Source: CAD feature listing. Evaluate the final solid. Frame: model axes, mm. A direction names the side the tool comes from. Coordinates: 2 decimals unless noted, no trailing zeros. Write each loop counter-clockwise with the first axis right and the second up, starting at its lowest first coordinate (ties: lowest second). Pieces come first, ordered by that corner, then holes. Notation, with made-up numbers: M 41,-36.5 L 66,-36.5 A18 ccw 66,-1.5 Z; hole C 38.5,62 d11. An arc over 180 degrees is marked long. Write item = value, one per line. Start each with the question number.
1. Access query for faces 1 (the face through (-9.65, 2.03, 2.3)), 2 (the face through (2.8, 7, 0)), 3 (the face through (6.5, -0.25, 6.37)), 4 (the face through (6.6, 0, -6.6)). Directions: +Z, -Z, +X, -X, +Y, -Y. A direction counts if a zero-diameter tool reaches every point of the face in a straight line with its end or side. Return the directions, or none.
2. Section query A-A (z = 0). Give the number of separate pieces and of enclosed holes in the cut face, then the cut area to 3 significant figures.
3. Pin query (flat end, axial travel): pin 1 Ø5 at (x, z) = (-11, 12) entering from -Y; pin 2 Ø5.5 at (x, z) = (12.5, 0) entering from -Y; pin 3 Ø2 at (y, z) = (4, 3.5) entering from -X; pin 4 Ø4 at (x, y) = (-5.5, 4) entering from -Z. Return the tip coordinate at first contact, or that it passes through.
4. Section query C-C (y = 3). Output: boundary loops of the cut face in (x, z).
5. Pull-direction query (Z, two-part tool) for faces 5 (the face through (-6.5, 0, -6.6)), 6 (the face through (2, 6, 13)), 7 (the face through (-7.12, 1.97, 7.02)); classes: pulls with the +Z half, pulls with the -Z half, needs draft (parallel to the pull), parting line crosses it, or undercut.
6. Line query: line 1 along Z through (x, y) = (0, 7.35); line 2 along X through (y, z) = (4.75, 2.5); line 3 along X through (y, z) = (5, -3). Output: solid intervals per line, ascending.
```python
from build123d import *

# Parameters (mm, degrees)
ESQUISSE1_R                  = 10
BOSS_EXTRU_1_DEPTH           = 4
ESQUISSE8_R                  = 11
BOSS_EXTRU_4_DEPTH           = 0.5
ESQUISSE3_R                  = 17.5
ESQUISSE3_R_2                = 1.7
BOSS_EXTRU_2_DEPTH           = 3.5
ENL_V_MAT_EXTRU_2_DEPTH      = 26.154522456
ENL_V_MAT_EXTRU_2_DEPTH_BACK = 1.5
ESQUISSE4_R                  = 3.55
ESQUISSE11_OUTSIDE_W         = 47.028
ESQUISSE11_OUTSIDE_H         = 47.028
ENL_V_MAT_EXTRU_3_DEPTH      = 27.009613607
CONG_1_R                     = 4
CONG_2_R                     = 1
CHANFREIN2_SIZE              = 0.4
ESQUISSE12_R                 = 1.7
ENL_V_MAT_EXTRU_4_DEPTH      = 27.009613773
ESQUISSE13_W                 = 5.6
ESQUISSE13_H                 = 5.6
ENL_V_MAT_EXTRU_5_DEPTH      = 2
BOSS_EXTRU_5_START           = 0.5
ESQUISSE14_R                 = 9.1
ESQUISSE14_R_2               = 1.7
BOSS_EXTRU_5_DEPTH           = 0.5
ESQUISSE15_R                 = 3.55
ENL_V_MAT_EXTRU_6_DEPTH      = 0.5


with BuildPart() as part:
    # Esquisse1 → Boss.-Extru.1 (new body)
    with BuildSketch(Plane(origin=(0, 0, 0), x_dir=(1, 0, 0), z_dir=(0, 1, 0))):
        with Locations(Location((0, 0, 0), (0, 0, 270))):
            Circle(ESQUISSE1_R)
    extrude(amount=BOSS_EXTRU_1_DEPTH)

    # Esquisse8 → Boss.-Extru.4 (add)
    with BuildSketch(Plane(origin=(0, 4, 0), x_dir=(1, 0, 0), z_dir=(0, 1, 0))):
        with Locations(Location((0, 0, 0), (0, 0, 270))):
            Circle(ESQUISSE8_R)
    extrude(amount=BOSS_EXTRU_4_DEPTH)

    # Esquisse3 → Boss.-Extru.2 (add)
    with BuildSketch(Plane(origin=(0, 4.5, 0), x_dir=(1, 0, 0), z_dir=(0, 1, 0))):
        with Locations(Location((0, 0, 0), (0, 0, 270))):
            Circle(ESQUISSE3_R)
        with Locations(Location((-12.5, 0, 0), (0, 0, 26.18008635))):
            Circle(ESQUISSE3_R_2, mode=Mode.SUBTRACT)
        with Locations(Location((0, 12.5, 0), (0, 0, 243.81991365))):
            Circle(ESQUISSE3_R_2, mode=Mode.SUBTRACT)
        with Locations(Location((12.5, 0, 0), (0, 0, 153.81991365))):
            Circle(ESQUISSE3_R_2, mode=Mode.SUBTRACT)
        with Locations(Location((0, -12.5, 0), (0, 0, 116.18008635))):
            Circle(ESQUISSE3_R_2, mode=Mode.SUBTRACT)
    extrude(amount=BOSS_EXTRU_2_DEPTH)

    # Esquisse4 → Enl_v. mat.-Extru.2 (cut, two sides: drawn at the far end of the back side and taken through both)
    with BuildSketch(Plane.XZ.offset(-4.5).offset(-ENL_V_MAT_EXTRU_2_DEPTH_BACK)):
        with Locations(Location((0, -12.5, 0), (0, 0, 129.122124479))):
            Circle(ESQUISSE4_R)
        with Locations(Location((-12.5, 0, 0), (0, 0, 57.371953872))):
            Circle(ESQUISSE4_R)
        with Locations(Location((0, 12.5, 0), (0, 0, 212.628046128))):
            Circle(ESQUISSE4_R)
        with Locations(Location((12.5, 0, 0), (0, 0, 122.628046128))):
            Circle(ESQUISSE4_R)
    extrude(amount=ENL_V_MAT_EXTRU_2_DEPTH + ENL_V_MAT_EXTRU_2_DEPTH_BACK, mode=Mode.SUBTRACT)

    # Esquisse11 outside → Enl_v. mat.-Extru.3 (cut, through all)
    with BuildSketch(Plane(origin=(0, 8, 0), x_dir=(1, 0, 0), z_dir=(0, 1, 0))):
        Rectangle(ESQUISSE11_OUTSIDE_W, ESQUISSE11_OUTSIDE_H)
        with BuildLine():
            ThreePointArc((-5.365249295, -11.29), (0, -18), (5.365249295, -11.29))
            ThreePointArc((5.365249295, -11.29), (8.838834765, -8.838834765), (11.29, -5.365249295))
            ThreePointArc((11.29, -5.365249295), (18, 0), (11.29, 5.365249295))
            ThreePointArc((11.29, 5.365249295), (8.838834765, 8.838834765), (5.365249295, 11.29))
            ThreePointArc((5.365249295, 11.29), (0, 18), (-5.365249295, 11.29))
            ThreePointArc((-5.365249295, 11.29), (-8.838834765, 8.838834765), (-11.29, 5.365249295))
            ThreePointArc((-11.29, 5.365249295), (-18, 0), (-11.29, -5.365249295))
            ThreePointArc((-11.29, -5.365249295), (-8.838834765, -8.838834765), (-5.365249295, -11.29))
        make_face(mode=Mode.SUBTRACT)
    extrude(amount=-ENL_V_MAT_EXTRU_3_DEPTH, mode=Mode.SUBTRACT)

    # Cong_1
    cong_1_edges = [part.edges().sort_by_distance(p)[0] for p in [
        (11.29, 6.25, -5.365249295),
        (5.365249295, 6.25, 11.29),
        (-11.29, 6.25, 5.365249295),
        (-5.365249295, 6.25, -11.29),
        (11.29, 6.25, 5.365249295),
        (-5.365249295, 6.25, 11.29),
        (-11.29, 6.25, -5.365249295),
        (5.365249295, 6.25, -11.29),
        (-2.702942841, 6.25, -17.29),
        (2.702942841, 6.25, -17.29),
        (-17.29, 6.25, 2.702942841),
        (-17.29, 6.25, -2.702942841),
        (2.702942841, 6.25, 17.29),
        (-2.702942841, 6.25, 17.29),
        (17.29, 6.25, -2.702942841),
        (17.29, 6.25, 2.702942841),
    ]]
    fillet(cong_1_edges, radius=CONG_1_R)

    # Cong_2
    # the kernel refuses this fillet: 1 mm, written as the material it takes off along each edge
    with BuildSketch(Plane(origin=(2.239962765, 4, -9.7459), x_dir=(0.968803091142529, 0, 0.24783173846922987), z_dir=(0, -1, 0)), Plane(origin=(-9.7459, 4, -2.239962765), x_dir=(0.24783173846923087, 0, -0.9688030911425286), z_dir=(0, -1, 0)), Plane(origin=(-2.239962765, 4, 9.7459), x_dir=(-0.9688030911425278, 0, -0.24783173846923437), z_dir=(0, -1, 0)), Plane(origin=(9.7459, 4, 2.239962765), x_dir=(-0.24783173846923068, 0, 0.9688030911425288), z_dir=(0, -1, 0))) as cong_2_piece_1:
        with BuildLine():
            CenterArc((0.465994929, 0.999699191), CONG_2_R, 223.166437968, 48.238942041)
            ThreePointArc((-0.263374559, 0.315579209), (-0.127115959, 0.161604715), (0, 0))
            ThreePointArc((0, 0), (0.245260489, -0.003008088), (0.490520978, 0))
        make_face()
    extrude(amount=5.226302444, mode=Mode.SUBTRACT)
    with BuildSketch(Plane(origin=(-2.239962765, 4, -9.7459), x_dir=(0.8110309236137252, 0, 0.5850032828474281), z_dir=(0, -1, 0)), Plane(origin=(9.7459, 4, -2.239962765), x_dir=(-0.5850032828485626, 0, 0.8110309236129067), z_dir=(0, -1, 0))) as cong_2_piece_2:
        with BuildLine():
            CenterArc((0.468936447, 0.998322771), CONG_2_R, 218.44215541, 48.238942041)
            ThreePointArc((-0.314299789, 0.376598556), (-0.15945936, 0.186371855), (0, 0))
            ThreePointArc((0, 0), (0.205521529, 0.005954162), (0.411043058, 0))
        make_face()
    extrude(amount=5.226302444, mode=Mode.SUBTRACT)
    with BuildSketch(Plane(origin=(-9.7459, 4, 2.239962765), x_dir=(0.2478317384692303, 0, 0.9688030911425288), z_dir=(0, -1, 0)), Plane(origin=(2.239962765, 4, 9.7459), x_dir=(0.9688030911425286, 0, -0.2478317384692314), z_dir=(0, -1, 0))) as cong_2_piece_3:
        with BuildLine():
            CenterArc((0.465994929, -0.999699191), CONG_2_R, 88.594619991, 48.238942041)
            ThreePointArc((-0.263374559, -0.315579209), (-0.127115959, -0.161604715), (0, 0))
            ThreePointArc((0, 0), (0.245260489, 0.003008088), (0.490520978, 0))
        make_face()
    extrude(amount=5.226302444, mode=Mode.SUBTRACT)

    # Chanfrein2
    chanfrein2_edges = [part.edges().sort_by_distance(p)[0] for p in [
        (-14.627830223, 8, -5.071719486),
        (8.838834765, 8, 8.838834765),
        (14.627830223, 8, 5.071719486),
        (17.5, 8, 0),
        (14.627830223, 8, -5.071719486),
        (8.838834765, 8, -8.838834765),
        (5.071719486, 8, -14.627830223),
        (0, 8, -17.5),
        (-5.071719486, 8, -14.627830223),
        (-8.838834765, 8, -8.838834765),
        (-17.5, 8, 0),
        (-14.627830223, 8, 5.071719486),
        (-8.838834765, 8, 8.838834765),
        (-5.071719486, 8, 14.627830223),
        (0, 8, 17.5),
        (5.071719486, 8, 14.627830223),
        (3.027485343, 8, 16.98773311),
        (-3.027485343, 8, 16.98773311),
        (16.98773311, 8, 3.027485343),
        (16.98773311, 8, -3.027485343),
        (3.027485343, 8, -16.98773311),
        (-3.027485343, 8, -16.98773311),
        (-16.98773311, 8, 3.027485343),
        (-16.98773311, 8, -3.027485343),
        (-11.490557352, 8, -6.002970096),
        (-6.002970096, 8, -11.490557352),
        (6.002970096, 8, -11.490557352),
        (11.490557352, 8, -6.002970096),
        (11.490557352, 8, 6.002970096),
        (6.002970096, 8, 11.490557352),
        (-11.490557352, 8, 6.002970096),
        (-6.002970096, 8, 11.490557352),
    ]]
    chamfer(chanfrein2_edges, length=CHANFREIN2_SIZE)

    # Esquisse12 → Enl_v. mat.-Extru.4 (cut, through all)
    with BuildSketch(Plane.XZ):
        with Locations(Location((0, 0, 0), (0, 0, 270))):
            Circle(ESQUISSE12_R)
    extrude(amount=-ENL_V_MAT_EXTRU_4_DEPTH, mode=Mode.SUBTRACT)

    # Esquisse13 → Enl_v. mat.-Extru.5 (cut)
    with BuildSketch(Plane(origin=(0, 8, 0), x_dir=(1, 0, 0), z_dir=(0, 1, 0))):
        Rectangle(ESQUISSE13_W, ESQUISSE13_H)
    extrude(amount=-ENL_V_MAT_EXTRU_5_DEPTH, mode=Mode.SUBTRACT)

    # Esquisse14 → Boss.-Extru.5 (add)
    with BuildSketch(Plane.XZ.offset(BOSS_EXTRU_5_START)):
        with Locations(Location((0, 0, 0), (0, 0, 84.512798049))):
            Circle(ESQUISSE14_R)
        with Locations(Location((0, 0, 0), (0, 0, 270))):
            Circle(ESQUISSE14_R_2, mode=Mode.SUBTRACT)
    extrude(amount=-BOSS_EXTRU_5_DEPTH)

    # Esquisse15 → Enl_v. mat.-Extru.6 (cut)
    with BuildSketch(Plane.XZ.offset(0.5)):
        with Locations(Location((12.5, 0, 0), (0, 0, 122.628046128))):
            Circle(ESQUISSE15_R)
        with Locations(Location((0, 12.5, 0), (0, 0, 212.628046128))):
            Circle(ESQUISSE15_R)
        with Locations(Location((-12.5, 0, 0), (0, 0, 57.371953872))):
            Circle(ESQUISSE15_R)
        with Locations(Location((0, -12.5, 0), (0, 0, 104.188876096))):
            Circle(ESQUISSE15_R)
    extrude(amount=-ENL_V_MAT_EXTRU_6_DEPTH, mode=Mode.SUBTRACT)


solid = part.part
```
Results are:
q1.face_1 = -X, -Y
q1.face_2 = +Y
q1.face_3 = +Z, +X, -Y
q1.face_4 = -Z, +X, -Y
q2.separate_pieces = 4
q2.enclosed_holes = 0
q2.area = 144 mm^2
q3.pin_1 = through
q3.pin_2 = 6
q3.pin_3 = -17.17
q3.pin_4 = -16.65
q4.outline = M -9.62,-2.72 A10 ccw -2.72,-9.62 A1 ccw -1.91,-9.51 A3.55 cw 1.91,-9.51 A1 ccw 2.72,-9.62 A10 ccw 9.62,-2.72 A1 ccw 9.51,-1.91 A3.55 cw 9.51,1.91 A1 ccw 9.62,2.72 A10 ccw 2.72,9.62 A1 ccw 1.91,9.51 A3.55 cw -1.91,9.51 A1 ccw -2.72,9.62 A10 ccw -9.62,2.72 A1 ccw -9.51,1.91 A3.55 cw -9.51,-1.91 A1 ccw Z; hole C 0,0 d3.4
q5.face_5 = needs draft
q5.face_6 = undercut
q5.face_7 = pulls with the +Z half
q6.line_1 = -17.5 to -14.2, -10.8 to -2.8, 2.8 to 10.8, 14.2 to 17.5
q6.line_2 = -17.22 to -15.02, -9.98 to 9.98, 15.02 to 17.22
q6.line_3 = -17 to -14.4, -10.6 to 10.6, 14.4 to 17
